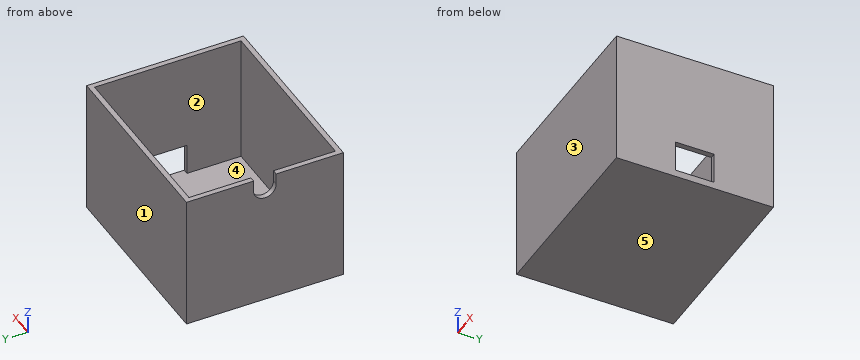
```python
from build123d import *

# Parameters (mm, degrees)
F0_W     = 55
F0_H     = 45
F1_DEPTH = 2
F2_W     = 55
F2_H     = 45
F2_W_2   = 51.9999974966
F2_H_2   = 41.9999974966
F3_DEPTH = 37
F5_DEPTH = 25
F6_W     = 11
F6_H     = 9
F7_DEPTH = 25


with BuildPart() as f1:
    # F0 (on Top) → F1 (new body)
    with BuildSketch(Plane.XY):
        with Locations((27.5, 22.5)):
            Rectangle(F0_W, F0_H)
    extrude(amount=F1_DEPTH)

    # F2 (on face) → F3 (join)
    with BuildSketch(Plane.XY.offset(2)):
        with Locations((27.5, 22.5)):
            Rectangle(F2_W, F2_H)
        with Locations((27.5, 22.5)):
            Rectangle(F2_W_2, F2_H_2, mode=Mode.SUBTRACT)
    extrude(amount=F3_DEPTH)

    # F4 (on face) → F5 (cut)
    with BuildSketch(Plane(origin=(0, 0, 0), x_dir=(0, -1, 0), z_dir=(-1, 0, 0))):
        with BuildLine():
            Line((-25.75, 39), (-25.75, 35.75))
            ThreePointArc((-25.75, 35.75), (-22.5, 32.5), (-19.25, 35.75))
            Line((-19.25, 35.75), (-19.25, 39))
            Line((-19.25, 39), (-25.75, 39))
        make_face()
    extrude(amount=-F5_DEPTH, mode=Mode.SUBTRACT)

    # F6 (on face) → F7 (cut)
    with BuildSketch(Plane.YZ.offset(55)):
        with Locations((22.5, 6.5)):
            Rectangle(F6_W, F6_H)
    extrude(amount=-F7_DEPTH, mode=Mode.SUBTRACT)


solid = f1.part
```
The listing builds one solid part. Answer for the finished solid, in the listing's coordinates (mm). Face numbers are marked on the shaded views. A direction names the side the tool comes from. Coordinates: 2 decimals unless noted, no trailing zeros. Loops run counter-clockwise (first coordinate to the right, second up) from the corner with the lowest first, then second, coordinate; pieces in that order, holes last. Notation, with made-up numbers: (-20.75, -22) -> (10.25, -22) arc R28 ccw to (10.25, 2) -> close; hole circle Ø2 at (-29.5, 2). An arc over 180 degrees is marked (long way). Return JSON: item names as keys, results as strings. Group by question number.
(1) Determine the mould class of the marked faces 3, 4 and 5 for opening direction Y: released by +Y, released by -Y, zero draft, split by the parting line, or undercut.
(2) A cutting plane is placed at B-B on z = 14.5. Write down the section's boundary in (x, y), and give its area (3 significant figures).
(3) Which of the six approach directions +Z, -Z, +X, -X, +Y, -Y give full straight-line access (tool end or side, diameter ignored) to the marked faces 1 and 2?
(4) A cutting plane is placed at D-D on y = 32.5. Write down the section's boundary in (x, z).
(5) A cutting plane is placed at A-A on y = 22.5. Write down the section's boundary in (x, z), and give its area (3 significant figures).
(6) Given pin 1 Ø2 at (x, y) = (48, 18) entering from +Z; pin 2 Ø1 at (y, z) = (25.5, 9) entering from +X, each flat-ended and moving along its own axis, determine where each tip first touches the part or whether it passes through.
(7) Find the intervals of material crossed by probe 1 along X at (y, z) = (14.5, 12); probe 2 along Y at (x, z) = (31.5, 7); probe 3 along Z at (x, y) = (18.5, 14), in increasing order. Write a range as from..to.
(8) A cutting plane is placed at C-C on x = 10.5. Write down the section's boundary in (y, z), and give its area (3 significant figures).
The answers:
{
 "1": {"face 3": "released by -Y", "face 4": "undercut", "face 5": "zero draft"},
 "2": {"outline": "(0, 0) -> (55, 0) -> (55, 45) -> (0, 45) -> close; hole (1.5, 1.5) -> (53.5, 1.5) -> (53.5, 43.5) -> (1.5, 43.5) -> close", "area": "291 mm^2"},
 "3": {"face 1": "+Z, -Z, +X, -X, +Y", "face 2": "+Z"},
 "4": {"outline": "(0, 0) -> (55, 0) -> (55, 39) -> (53.5, 39) -> (53.5, 2) -> (1.5, 2) -> (1.5, 39) -> (0, 39) -> close"},
 "5": {"outline": "(0, 0) -> (55, 0) -> (55, 2) -> (1.5, 2) -> (1.5, 32.5) -> (0, 32.5) -> close; (53.5, 11) -> (55, 11) -> (55, 39) -> (53.5, 39) -> close", "area": "198 mm^2"},
 "6": {"pin 1": "stops at z = 2", "pin 2": "stops at x = 1.5"},
 "7": {"probe 1": "x = 0..1.5, 53.5..55", "probe 2": "y = 0..1.5, 43.5..45", "probe 3": "z = 0..2"},
 "8": {"outline": "(0, 0) -> (45, 0) -> (45, 39) -> (43.5, 39) -> (43.5, 2) -> (1.5, 2) -> (1.5, 39) -> (0, 39) -> close", "area": "201 mm^2"}
}
